Read the model definition and answer for the solid it produces. Units are mm, in the model's axes. A direction names the side the tool comes from. Coordinates: 2 decimals unless noted, no trailing zeros. Write each loop counter-clockwise with the first axis right and the second up, starting at its lowest first coordinate (ties: lowest second). Pieces come first, ordered by that corner, then holes.
(1) The part is cut by section A-A, the plane x = 6.5. Determine the outline of the cut face in (y, z).
(2) The part is cut by section C-C, the plane y = 48.85. Determine the outline of the cut face in (x, z), and give its area (3 significant figures).
(3) Straight lines are drawn through the part: line 1 along Y through (x, z) = (8.3, 0); line 2 along Z through (x, y) = (9, 0); line 3 along Y through (x, z) = (2, 0). For each, find the intervals that lie inside material, in ascending order.
(4) Determine the mould class of faces 1 (the flat face through (-1, -3, -21)), 2 (the flat face through (-8, 0, 20)), 3 (the cylindrical face through (2.46, 53.24, 0.98)) for opening direction Z: pulls with the +Z half, pulls with the -Z half, needs draft (parallel to the pull), parting line crosses it, or undercut.
(5) The part is cut by section B-B, the plane x = -9. Determine the outline of the cut face in (y, z), and give its area (3 significant figures).
(6) The part is cut by section D-D, the plane x = -1. Determine the outline of the cut face in (y, z), and give its area (3 significant figures).
(7) Given pin 1 (8 mm diameter, centred on y = 41, z = -2.5, fed in from -X); pin 2 (5 mm diameter, centred on y = 0, z = 12.5, fed in from +X); pin 3 (1.6 mm diameter, centred on y = -4.5, z = -21.5, fed in from -X), each flat-ended and moving along its own axis, determine where each tip first touches the part or whether it passes through.
(8) Which of the six approach directions +Z, -Z, +X, -X, +Y, -Y give full straight-line access (tool end or side, diameter ignored) to faces 4 (the flat face through (-9, 1, 12.5)), 5 (the cylindrical face through (6.08, 2.23, -0.29)), 6 (the flat face through (5, 66, 2)), 7 (the flat face through (-8, 7.5, -19))?
```python
from build123d import *

# Parameters (mm, degrees)
BOSS_EXTRUDE1_DEPTH            = 7.5
CBORE_FOR_M3_SHCS1_AT_2_COUNT  = 2
CBORE_FOR_M3_SHCS1_AT_2_PITCH  = 7.5
FILLET1_R                      = 3
CBORE_FOR_M3_SHCS2_D           = 4.5
CBORE_FOR_M3_SHCS2_DEPTH       = 7
CBORE_FOR_M3_SHCS2_CBORE_D     = 5.5
CBORE_FOR_M3_SHCS2_CBORE_DEPTH = 0.75
CBORE_FOR_M3_SHCS2_TIP         = 1.351936393
SKETCH9_W                      = 15
SKETCH9_H                      = 62.5
BOSS_EXTRUDE2_DEPTH            = 10
CBORE_FOR_M5_SHCS1_D           = 5.5
CBORE_FOR_M5_SHCS1_DEPTH       = 15
CBORE_FOR_M5_SHCS1_CBORE_D     = 9
CBORE_FOR_M5_SHCS1_CBORE_DEPTH = 5
CBORE_FOR_M5_SHCS1_TIP         = 1.652366702
SKETCH12_W                     = 22.5
SKETCH12_H                     = 2
BOSS_EXTRUDE3_DEPTH            = 3
FILLET2_R                      = 10
FILLET3_R                      = 2.5


with BuildPart() as part:
    # Sketch1 → Boss-Extrude1 (new, symmetric)
    with BuildSketch(Plane(origin=(0, 0, 0), x_dir=(1, 0, 0), z_dir=(0, 1, 0))):
        Polygon((0, 12.5), (0, -12.5), (-15.5, -12.5), (-15.5, -11.829), (-26.247516559, -17.166685624), (-26.247516559, -20), (10, -20), (10, 20), (-26.247516559, 20), (-26.247516559, 17.166685624), (-15.5, 11.829), (-15.5, 12.5), align=None)
    extrude(amount=BOSS_EXTRUDE1_DEPTH, both=True)

    # Sketch4 → CBORE for M3 SHCS1 (revolve, cut)
    with BuildSketch(Plane(origin=(-20.873758279, 3.75, -14.497842812), x_dir=(0.8956263799062305, 0, 0.4448071353025496), z_dir=(0, 1, 0))):
        Polygon((0, 0), (0, 18.6607451), (3, 18.6607451), (3, 3), (1.625, 3), (1.625, 0), align=None)
    cbore_for_m3_shcs1 = revolve(axis=Axis((-23.698283589, 3.75, -8.810615299), (0.44480713530254956, 0, -0.8956263799062304)), mode=Mode.SUBTRACT)

    # CBORE for M3 SHCS1 at 2: CBORE for M3 SHCS1 ×2
    with Locations(*[(0, -i * CBORE_FOR_M3_SHCS1_AT_2_PITCH, 0) for i in range(1, CBORE_FOR_M3_SHCS1_AT_2_COUNT)]):
        add(cbore_for_m3_shcs1, mode=Mode.SUBTRACT)

    # Mirror1: CBORE for M3 SHCS1 across plane
    add(cbore_for_m3_shcs1.mirror(Plane.XY), mode=Mode.SUBTRACT)

    # Mirror1 copy 1 sketch → Mirror1 copy 1 (revolve, cut)
    with BuildSketch(Plane(origin=(-20.873758279, -3.75, 14.497842812), x_dir=(0.8956263799062305, 0, -0.4448071353025496), z_dir=(0, 1, 0))):
        Polygon((0, 0), (0, -18.6607451), (3, -18.6607451), (3, -3), (1.625, -3), (1.625, 0), align=None)
    revolve(axis=Axis((-23.698283589, -3.75, 8.810615299), (-0.44480713530254956, 0, -0.8956263799062304)), mode=Mode.SUBTRACT)

    # Fillet1
    fillet1_edges = [part.edges().sort_by_distance(p)[0] for p in [
        (0, 0, 12.5),
        (0, 0, -12.5),
    ]]
    fillet(fillet1_edges, radius=FILLET1_R)

    # CBORE for M3 SHCS2
    with Locations(Plane(origin=(10, 0, 0), x_dir=(0, 0, -1), z_dir=(1, 0, 0))):
        with Locations((-12.5, 0), (0, 0), (12.5, 0)):
            CounterBoreHole(CBORE_FOR_M3_SHCS2_D / 2, CBORE_FOR_M3_SHCS2_CBORE_D / 2, CBORE_FOR_M3_SHCS2_CBORE_DEPTH, depth=CBORE_FOR_M3_SHCS2_DEPTH)
            with Locations((0, 0, -(CBORE_FOR_M3_SHCS2_DEPTH + CBORE_FOR_M3_SHCS2_TIP / 2))):  # 118° drill point
                Cone(0, CBORE_FOR_M3_SHCS2_D / 2, CBORE_FOR_M3_SHCS2_TIP, mode=Mode.SUBTRACT)

    # Sketch9 → Boss-Extrude2 (add)
    with BuildSketch(Plane(origin=(10, 0, 0), x_dir=(0, 0, -1), z_dir=(1, 0, 0))):
        with Locations((0, 38.75)):
            Rectangle(SKETCH9_W, SKETCH9_H)
    extrude(amount=-BOSS_EXTRUDE2_DEPTH)

    # CBORE for M5 SHCS1
    with Locations(Plane(origin=(0, 0, 0), x_dir=(0, 0, -1), z_dir=(-1, 0, 0))):
        with Locations((0, -63.85), (0, -48.85)):
            CounterBoreHole(CBORE_FOR_M5_SHCS1_D / 2, CBORE_FOR_M5_SHCS1_CBORE_D / 2, CBORE_FOR_M5_SHCS1_CBORE_DEPTH, depth=CBORE_FOR_M5_SHCS1_DEPTH)
            with Locations((0, 0, -(CBORE_FOR_M5_SHCS1_DEPTH + CBORE_FOR_M5_SHCS1_TIP / 2))):  # 118° drill point
                Cone(0, CBORE_FOR_M5_SHCS1_D / 2, CBORE_FOR_M5_SHCS1_TIP, mode=Mode.SUBTRACT)

    # Sketch12 → Boss-Extrude3 (add)
    with BuildSketch(Plane(origin=(0, 0, -20), x_dir=(-1, 0, 0), z_dir=(0, 0, -1))):
        with Locations((1.25, -4)):
            Rectangle(SKETCH12_W, SKETCH12_H)
    extrude(amount=BOSS_EXTRUDE3_DEPTH)

    # Fillet2
    fillet2_edges = [part.edges().sort_by_distance(p)[0] for p in [
        (5, 7.5, -7.5),
        (5, 7.5, 7.5),
    ]]
    fillet(fillet2_edges, radius=FILLET2_R)

    # Fillet3
    fillet3_edges = [part.edges().sort_by_distance(p)[0] for p in [
        (5, 70, -7.5),
        (5, 70, 7.5),
    ]]
    fillet(fillet3_edges, radius=FILLET3_R)


solid = part.part
```
Computed:
1. outline: (-7.5, -20) - (-5, -20) - (-5, -23) - (-3, -23) - (-3, -20) - (7.5, -20) - (7.5, -17.5) arc R10 cw to (17.5, -7.5) - (67.5, -7.5) arc R2.5 ccw to (70, -5) - (70, 5) arc R2.5 ccw to (67.5, 7.5) - (17.5, 7.5) arc R10 cw to (7.5, 17.5) - (7.5, 20) - (-7.5, 20) - close; hole circle Ø4.5 at (0, -12.5); hole circle Ø4.5 at (0, 0); hole circle Ø4.5 at (0, 12.5); hole circle Ø5.5 at (48.85, 0); hole circle Ø5.5 at (63.85, 0)
2. outline: (0, -7.5) - (10, -7.5) - (10, -2.75) - (5, -2.75) - (5, -4.5) - (0, -4.5) - close; (0, 4.5) - (5, 4.5) - (5, 2.75) - (10, 2.75) - (10, 7.5) - (0, 7.5) - close
2. area: 77.5 mm2
3. line 1: y = -7.5 to -2.25, 2.25 to 46.1, 51.6 to 61.1, 66.6 to 70
3. line 2: z = -20 to -14.75, -10.25 to -2.25, 2.25 to 10.25, 14.75 to 20
3. line 3: y = -7.5 to -0.59, 0.59 to 44.35, 53.35 to 59.35, 68.35 to 70
4. face 1: needs draft
4. face 2: pulls with the +Z half
4. face 3: undercut
5. outline: (-7.5, -20) - (-5, -20) - (-5, -23) - (-3, -23) - (-3, -20) - (7.5, -20) - (7.5, -17.5) arc R10 cw to (8.84, -12.5) - (-7.5, -12.5) - close; (-7.5, 12.5) - (8.84, 12.5) arc R10 cw to (7.5, 17.5) - (7.5, 20) - (-7.5, 20) - close
5. area: 235 mm2
6. outline: (-7.5, -20) - (-5, -20) - (-5, -23) - (-3, -23) - (-3, -20) - (7.5, -20) - (7.5, -17.5) arc R10 cw to (9.33, -11.74) - (-7.5, -11.74) - close; (-7.5, 11.74) - (9.33, 11.74) arc R10 cw to (7.5, 17.5) - (7.5, 20) - (-7.5, 20) - close
6. area: 261 mm2
7. pin 1: stops at x = 0
7. pin 2: stops at x = 9.25
7. pin 3: stops at x = -12.5
8. face 4: +Y, -Y
8. face 5: +X
8. face 6: -X
8. face 7: -Z, +X, -X, +Y
